from build123d import *

# Parameters (mm, degrees)
F0_R            = 15
F2_DEPTH        = 8
F5_COPIES_COUNT = 3
F6_R            = 3.99999
F7_R            = 1.5
F9_DEPTH        = 25


# Not quite as in the source:
# - a fillet or chamfer is up to 0.001 mm smaller than in the source, because OpenCascade refuses the exact size
# - a pattern or mirror of a feature is missing from the dataset's text; its kind, count and spacing are read off the source's solid


with BuildPart() as f2:
    # F0 (on Top) → F2 (new body)
    with BuildSketch(Plane.XY):
        with BuildLine():
            Line((-5.5, 23.6913686675), (-5.5, 19.228884523))
            ThreePointArc((-5.5, 19.228884523), (-17.3205080757, 10), (-19.4027024834, -4.8513025407))
            Line((-19.4027024834, -4.8513025407), (-23.2673271165, -7.0825446129))
            Line((-23.2673271165, -7.0825446129), (-22.2673271165, -8.8145954205))
            Line((-22.2673271165, -8.8145954205), (-18.8032255014, -6.8145954205))
            ThreePointArc((-18.8032255014, -6.8145954205), (-16.0775588327, -9.28238292), (-15.3032255014, -12.876773247))
            Line((-15.3032255014, -12.876773247), (-18.7673271165, -14.876773247))
            Line((-18.7673271165, -14.876773247), (-17.7673271165, -16.6088240546))
            Line((-17.7673271165, -16.6088240546), (-13.9027024834, -14.3775819823))
            ThreePointArc((-13.9027024834, -14.3775819823), (0, -20), (13.9027024834, -14.3775819823))
            Line((13.9027024834, -14.3775819823), (17.7673271165, -16.6088240546))
            Line((17.7673271165, -16.6088240546), (18.7673271165, -14.876773247))
            Line((18.7673271165, -14.876773247), (15.3032255014, -12.876773247))
            ThreePointArc((15.3032255014, -12.876773247), (16.0775588327, -9.28238292), (18.8032255014, -6.8145954205))
            Line((18.8032255014, -6.8145954205), (22.2673271165, -8.8145954205))
            Line((22.2673271165, -8.8145954205), (23.2673271165, -7.0825446129))
            Line((23.2673271165, -7.0825446129), (19.4027024834, -4.8513025407))
            ThreePointArc((19.4027024834, -4.8513025407), (17.3205080757, 10), (5.5, 19.228884523))
            Line((5.5, 19.228884523), (5.5, 23.6913686675))
            Line((5.5, 23.6913686675), (3.5, 23.6913686675))
            Line((3.5, 23.6913686675), (3.5, 19.6913686675))
            ThreePointArc((3.5, 19.6913686675), (0, 18.5647658399), (-3.5, 19.6913686675))
            Line((-3.5, 19.6913686675), (-3.5, 23.6913686675))
            Line((-3.5, 23.6913686675), (-5.5, 23.6913686675))
        make_face()
        Circle(F0_R, mode=Mode.SUBTRACT)
    extrude(amount=F2_DEPTH)

    # F4 (on offset) → F5 (revolve, cut)
    with BuildSketch(Plane.XY.offset(4)):
        with BuildLine():
            Line((0, 17.1913686675), (0, 25.3913686675))
            ThreePointArc((0, 25.3913686675), (-4.1, 21.2913686675), (0, 17.1913686675))
        make_face()
    f5 = revolve(axis=Axis((0, 21.2913686675, 4), (0, -1, 0)), mode=Mode.SUBTRACT)

    # F5_copies: F5 ×3 about axis
    f5_copies_axis = Axis((0, 0, 0), (0, 0, 1))
    for i in range(1, F5_COPIES_COUNT):
        add(f5.rotate(f5_copies_axis, i * 360 / F5_COPIES_COUNT), mode=Mode.SUBTRACT)

    # F6 (radius 4 in the source; OpenCascade refuses exactly that, so slightly less here)
    f6_edges = [f2.edges().sort_by_distance(p)[0] for p in [
        (-4.5, 23.691369, 8),
        (4.5, 23.691369, 8),
        (22.767327, -7.94857, 8),
        (18.267327, -15.742799, 8),
        (-18.267327, -15.742799, 8),
        (-22.767327, -7.94857, 8),
        (-18.267327, -15.742799, 0),
        (-22.767327, -7.94857, 0),
        (18.267327, -15.742799, 0),
        (22.767327, -7.94857, 0),
        (4.5, 23.691369, 0),
        (-4.5, 23.691369, 0),
    ]]
    fillet(f6_edges, radius=F6_R)

    # F7
    f7_edges = [f2.edges().sort_by_distance(p)[0] for p in [
        (-19.402702, -4.851303, 4),
        (-5.5, 19.228885, 4),
        (5.5, 19.228885, 4),
        (19.402702, -4.851303, 4),
        (13.902702, -14.377582, 4),
        (-13.902702, -14.377582, 4),
    ]]
    fillet(f7_edges, radius=F7_R)

    # F8 (on face) → F9 (join)
    with BuildSketch(Plane.XY.offset(8)):
        Polygon((-10.5356537529, 17), (-13.2287565553, 15), (-1.63e-08, 15), (13.2287565553, 15), (10.5356537529, 17), align=None)
        Polygon((13.2287565553, -15), (0, -15), (-13.2287565553, -15), (-10.5356537529, -17), (10.5356537529, -17), align=None)
    extrude(amount=F9_DEPTH)


solid = f2.part
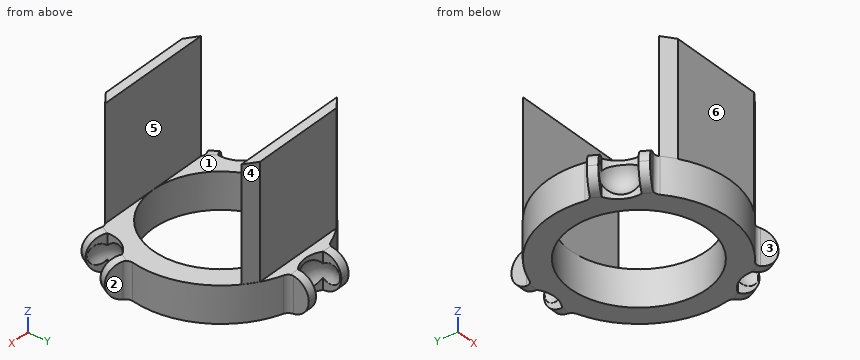
Part model, mm, in its own coordinate system. Face numbers are marked on the shaded views. A direction names the side the tool comes from. Round coordinates to 2 decimals unless told otherwise and drop trailing zeros. Write each loop counter-clockwise with the first axis right and the second up, starting at its lowest first coordinate (ties: lowest second). Pieces come first, ordered by that corner, then holes. Notation, with made-up numbers: M -35,72.25 L -5,72.25 A14 cw -5,86.25 Z; hole C -10.75,-9 d10. An arc over 180 degrees is marked long. Return JSON: item names as keys, results as strings. Group by question number.
(1) Saw through at B-B on z = 19. Write the cut outline in (x, y).
(2) Saw through at A-A on y = 0. Write the cut outline in (x, z).
(3) Drill centre lines: probe 1 along X at (y, z) = (0, 5.5); probe 2 along Y at (x, z) = (0, 4); probe 3 along Z at (x, y) = (16.5, 5). Where is each one in solid material? Low to high.
(4) Saw through at D-D on y = -11. Write the cut outline in (x, z).
(5) Pin check, flat tips, straight feed: pin 1 Ø10 at (x, y) = (8.5, 8) entering from +Z; pin 2 Ø17 at (x, z) = (1, 19) entering from +Y; pin 3 Ø8 at (y, z) = (4.5, 14) entering from +X; pin 4 Ø2.5 at (y, z) = (22, 6) entering from +X. Stop position of each tip, or through.
(6) Which spindle directions (+Z, -Z, +X, -X, +Y, -Y) get a long thin tool onto all of the face, cutting with end or side? Do the marked faces 4, 5 and 6. Say none if no direction does.
(7) Two-plate mould, pull along X, no slides. Class the marked faces 1, 2 and 3: +X half, -X half, draft (parallel to the pull), parting line (faces both ways), or undercut.
(8) Saw through at C-C on x = 9. Write the cut outline in (y, z).
Returned:
{
 "1": {"outline": "M -13.23,-15 L -10.54,-17 L 10.54,-17 L 13.23,-15 Z; M -13.23,15 L 13.23,15 L 10.54,17 L -10.54,17 Z"},
 "2": {"outline": "M -20,0 L -15,0 L -15,8 L -20,8 Z; M 15,0 L 20,0 L 20,8 L 15,8 Z"},
 "3": {"probe 1": "-20 to -15, 15 to 20", "probe 2": "-20 to -15, 15 to 17.19", "probe 3": "0 to 8"},
 "4": {"outline": "M -15.41,0 L -10.2,0 L -10.2,8 L -15.41,8 L -15.41,6.74 A4.08 cw -15.41,1.26 Z; M 10.2,0 L 15.41,0 L 15.41,1.26 A4.08 cw 15.41,6.74 L 15.41,8 L 10.2,8 Z"},
 "5": {"pin 1": "z = 8", "pin 2": "y = 17", "pin 3": "through", "pin 4": "x = 5.5"},
 "6": {"face 4": "+Z, +X, +Y", "face 5": "+Z, +X, -X", "face 6": "+Z, +X, -X, -Y"},
 "7": {"face 1": "draft", "face 2": "+X half", "face 3": "undercut"},
 "8": {"outline": "M -17.86,0 L -12,0 L -12,8 L -15,8 L -15,33 L -17,33 L -17,8 L -17.86,8 Z; M 12,0 L 17.86,0 L 17.86,8 L 17,8 L 17,33 L 15,33 L 15,8 L 12,8 Z"}
}
